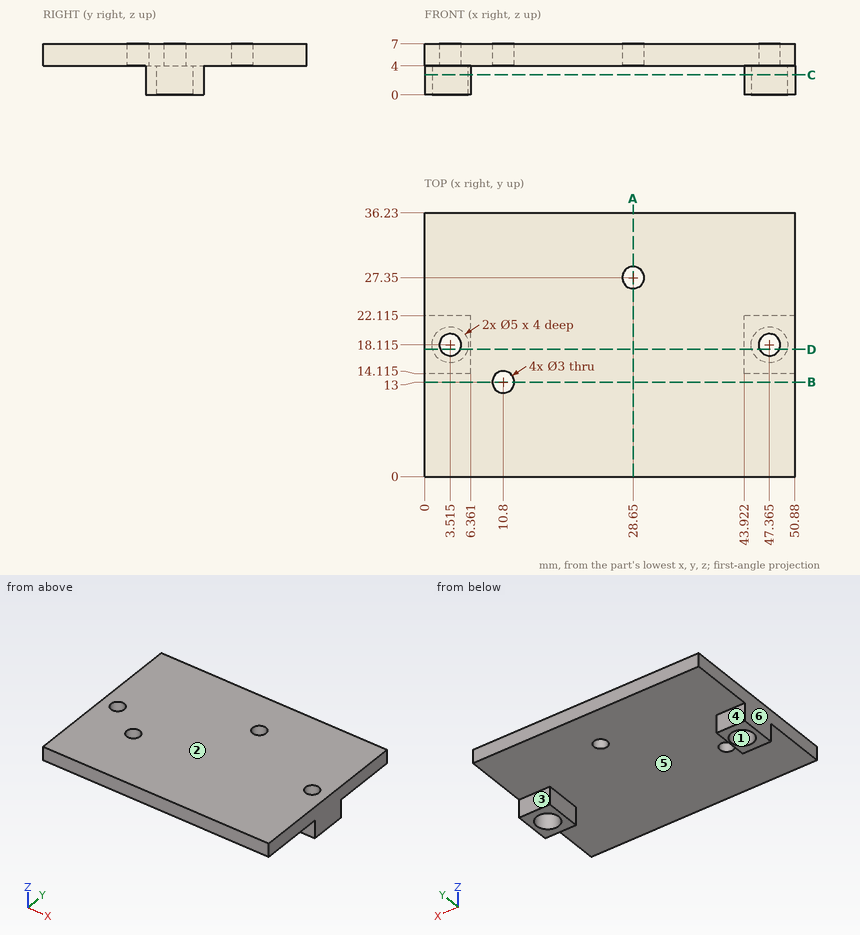
Could you check a few things on this drawing? It's one solid part, dimensions in mm from its lowest x, y, z. A direction names the side the tool comes from. Give positions to 0.01 mm unless a question says otherwise; leave off trailing zeros. Loops run counter-clockwise (first coordinate to the right, second up) from the corner with the lowest first, then second, coordinate; pieces in that order, holes last. Notation, with made-up numbers: M 14.5,-10 L 36.5,-10 A17 ccw 36.5,-5 Z; hole C 37,89 d5. An arc over 180 degrees is marked long. Answer as a JSON object with one key per item and string values.
Q1. Suppose I cut it at B-B, the plane y = 13. List the corners of the cut face in (x, z) for me, plus the area to 3 significant figures.
Values found:
{"outline": "M 0,4 L 9.3,4 L 9.3,7 L 0,7 Z; M 12.3,4 L 50.88,4 L 50.88,7 L 12.3,7 Z", "area": "144 mm²"}
Q2. Suppose I cut it at D-D, the plane y = 17.5. List the corners of the cut face in (x, z) for me, plus the area to 3 significant figures.
Values found:
{"outline": "M 0,0 L 1.09,0 L 1.09,4 L 2.15,4 L 2.15,7 L 0,7 Z; M 4.88,4 L 5.94,4 L 5.94,0 L 6.36,0 L 6.36,4 L 43.92,4 L 43.92,0 L 44.94,0 L 44.94,4 L 46,4 L 46,7 L 4.88,7 Z; M 48.73,4 L 49.79,4 L 49.79,0 L 50.88,0 L 50.88,7 L 48.73,7 Z", "area": "151 mm²"}
Q3. For P1, Ø4, axis at x = 28.65, y = 27.35, coming from the -Z side; P2, Ø1.8, axis at x = 47.365, y = 18.115, coming from the +Z side; P3, Ø6.5, axis at x = 3.515, y = 18.115, coming from the -Z side; P4, Ø2, axis at x = 2, z = 2.5, coming from the +Y side (1 decimal), each with a flat end and sliding along its axis, tell me the tip position at first contact or that it passes through.
Values found:
{"P1": "stops at z = 4", "P2": "passes through", "P3": "stops at z = 0", "P4": "stops at y = 22.1"}
Q4. For the marked faces 1, 2 and 3, which set-ups out of +Z, -Z, +X, -X, +Y, -Y let a thin tool reach every point of the face, with its end or its side?
Values found:
{"face 1": "-Z", "face 2": "+Z, +X, -X, +Y, -Y", "face 3": "-Z, +X, -X, +Y"}
Q5. Suppose I cut it at A-A, the plane x = 28.65. List the corners of the cut face in (y, z) for me.
Values found:
{"outline": "M 0,4 L 25.85,4 L 25.85,7 L 0,7 Z; M 28.85,4 L 36.23,4 L 36.23,7 L 28.85,7 Z"}
Q6. If we mould it in two halves opening along X, with no side actions, what happens to the marked faces 4, 5 and 6? For each: pulls with the +X half, pulls with the -X half, needs draft (parallel to the pull), parting line crosses it, or undercut.
Values found:
{"face 4": "needs draft", "face 5": "undercut", "face 6": "pulls with the -X half"}
Q7. If I drill on probe 1 along Z at (x, y) = (47.5, 7.5); probe 2 along X at (y, z) = (22, 3.75); probe 3 along Y at (x, z) = (10.8, 5.05), over which ranges is the centre line in solid material (lowest first)? Write a range as [from, to].
Values found:
{"probe 1": "z = [4, 7]", "probe 2": "x = [0, 6.36], [43.92, 50.88]", "probe 3": "y = [0, 11.5], [14.5, 36.23]"}
Q8. Suppose I cut it at C-C, the plane z = 2.75. List the corners of the cut face in (x, y) for me (1 decimal).
Values found:
{"outline": "M 0,14.1 L 6.4,14.1 L 6.4,22.1 L 0,22.1 Z; M 43.9,14.1 L 50.9,14.1 L 50.9,22.1 L 43.9,22.1 Z; hole C 3.5,18.1 d5; hole C 47.4,18.1 d5"}
